Build history of the part. All positions in model axes, mm. A direction names the side the tool comes from. Give positions to 0.01 mm unless a question says otherwise; leave off trailing zeros. Loops run counter-clockwise (first coordinate to the right, second up) from the corner with the lowest first, then second, coordinate; pieces in that order, holes last. Notation, with made-up numbers: M 84,89.5 L 121,89.5 A20 cw 121,100.5 Z; hole C -1.75,-11 d9. An arc over 180 degrees is marked long. Put each result on its own line as item: value.
Autodesk Inventor part; units mm, degrees
ref_plane "作業平面1" through (-10, -78.5, 30.5) normal (0, 0, -1) x (0, 1, 0)
ref_plane "YZ Plane" through (0, 0, 0) normal (1, 0, 0) x (0, 1, 0)
ref_plane "XZ Plane" through (0, 0, 0) normal (0, 1, 0) x (-1, 0, 0)
sketch "スケッチ1" plane through (0, 0, 0) normal (0, 0, 1) x (1, 0, 0)
  circle A0 centre (7, -1.5) radius 1.1
  circle A1 centre (-7, -1.5) radius 1.1
  arc A2 (-7, 6.5) -> (-4, 3.5) centre (-4, 6.5) ccw
  line L0 (4, 3.5) -> (-4, 3.5)
  arc A3 (4, 3.5) -> (7, 6.5) centre (4, 6.5) ccw
  line L1 (7, 27.5) -> (7, 6.5)
  line L2 (-7, 6.5) -> (-7, 27.5)
  arc A4 (-4, 30.5) -> (-7, 27.5) centre (-4, 27.5) ccw
  line L3 (-4, 30.5) -> (4, 30.5)
  circle A5 centre (-7, 35.5) radius 1.1
  circle A6 centre (7, 35.5) radius 1.1
  circle A7 centre (-7, -1.5) radius 1.1
  line L4 (7, 27.5) -> (7, 6.5)
  arc A8 (4, 3.5) -> (7, 6.5) centre (4, 6.5) ccw
  line L5 (4, 3.5) -> (-4, 3.5)
  arc A9 (-7, 6.5) -> (-4, 3.5) centre (-4, 6.5) ccw
  line L6 (-7, 6.5) -> (-7, 27.5)
  arc A10 (-4, 30.5) -> (-7, 27.5) centre (-4, 27.5) ccw
  line L7 (-4, 30.5) -> (4, 30.5)
  arc A11 (7, 27.5) -> (4, 30.5) centre (4, 27.5) ccw
  circle A12 centre (7, -1.5) radius 1.1
  arc A13 (6, -30) -> (6.4, -31.2) centre (8, -30) ccw
  arc A14 (6.4, -40.8) -> (6.4, -31.2) centre (0, -36) ccw
  arc A15 (6.4, -40.8) -> (6, -42) centre (8, -42) ccw
  line L8 (6, -42) -> (6, -42.5)
  arc A16 (6, -42.5) -> (10, -42.5) centre (8, -42.5) ccw
  line L9 (10, -42.5) -> (10, 76.5)
  arc A17 (10, 76.5) -> (6, 76.5) centre (8, 76.5) ccw
  line L10 (6, 76.5) -> (6, 76)
  arc A18 (6, 76) -> (6.4, 74.8) centre (8, 76) ccw
  arc A19 (6.4, 65.2) -> (6.4, 74.8) centre (0, 70) ccw
  arc A20 (6.4, 65.2) -> (6, 64) centre (8, 64) ccw
  line L11 (6, 64) -> (6, 60.696)
  arc A21 (6, 60.696) -> (6.9906, 58.9694) centre (8, 60.696) ccw
  line L12 (6.9906, 58.9694) -> (6.9906, 52.6121)
  arc A22 (6.9906, 52.6121) -> (6, 50.8855) centre (8, 50.8855) ccw
  line L13 (6, 50.8855) -> (6, 45.5)
  arc A23 (3, 42.5) -> (6, 45.5) centre (3, 45.5) ccw
  line L14 (3, 42.5) -> (-8, 42.5)
  arc A24 (-8, 42.5) -> (-10, 40.5) centre (-8, 40.5) ccw
  line L15 (-10, 40.5) -> (-10, -6.5)
  arc A25 (-10, -6.5) -> (-8, -8.5) centre (-8, -6.5) ccw
  line L16 (-8, -8.5) -> (3, -8.5)
  arc A26 (6, -11.5) -> (3, -8.5) centre (3, -11.5) ccw
  line L17 (6, -11.5) -> (6, -16.8855)
  arc A27 (6, -16.8855) -> (6.9906, -18.6121) centre (8, -16.8855) ccw
  line L18 (6.9906, -18.6121) -> (6.9906, -24.9694)
  arc A28 (6.9906, -24.9694) -> (6, -26.696) centre (8, -26.696) ccw
  line L19 (6, -26.696) -> (6, -30)
  circle A29 centre (8, 76.5) radius 1.1
  circle A30 centre (-8, 40.5) radius 1.1
  circle A31 centre (-8, -6.5) radius 1.1
  circle A32 centre (8, -42.5) radius 1.1
  circle A33 centre (8, -6.5) radius 1.1
  circle A34 centre (8, 40.5) radius 1.1
  line L20 (10, 37.6) -> (-10, 37.6)
  line L21 (10, 17) -> (-10, 17) construction
  line L22 (10, -3.6) -> (-10, -3.6)
  point P0 (0, 0)
  point P1 (-10, -3.6)
  point P2 (10, -3.6)
  dimension "d0" = 1
ref_plane "作業平面1" through (-10, -78.5, 30.5) normal (0, 0, -1) x (0, 1, 0)
extrude "押し出し1" add sketch "スケッチ1" along normal up to surface (30.5 mm away) contours L22 L15 L20 L9
fillet "フィレット1" radius 4.25 4 edges at (10, 37.6, 15.25) (-10, 37.6, 15.25) (10, -3.6, 15.25) (-10, -3.6, 15.25)
properties part number "suzikai" material "ABS プラスチック"
Q1. Drop a flat-ended pin along its axis: pin 1 Ø3 at (x, y) = (7, -1.5) entering from +Z. Give the stop position or say it passes through.
Here are the results:
pin 1: z = 30.5
Q2. Mould opens along X. For faces 3 (the flat face through (0, 37.6, 15)), 4 (the cylindrical face through (-8.79, -2.32, 15.46)), 5 (the cylindrical face through (-6.1, 4.36, 15.04)), 6 (the flat face through (10, 17, 15)) say: pulls with the +X half, pulls with the -X half, needs draft (parallel to the pull), parting line crosses it, or undercut.
Here are the results:
face 3: needs draft
face 4: pulls with the -X half
face 5: undercut
face 6: pulls with the +X half
Q3. Slice it at A-A (x = 2.5). List the corners of the cut face in (y, z), and give its area (3 significant figures).
Here are the results:
outline: M -3.6,0 L 3.5,0 L 3.5,30.5 L -3.6,30.5 Z; M 30.5,0 L 37.6,0 L 37.6,30.5 L 30.5,30.5 Z
area: 433 mm²
Q4. Slice it at D-D (x = 6.5). List the corners of the cut face in (y, z).
Here are the results:
outline: M -3.53,0 L -2.48,0 L -2.48,30.5 L -3.53,30.5 Z; M -0.52,0 L 4.84,0 L 4.84,30.5 L -0.52,30.5 Z; M 29.16,0 L 34.52,0 L 34.52,30.5 L 29.16,30.5 Z; M 36.48,0 L 37.53,0 L 37.53,30.5 L 36.48,30.5 Z
Q5. Probe line 1 (X direction, y = 17.5, z = 25); line 2 (X direction, y = -1, z = 22); line 3 (Y direction, x = -8, z = 20). List the from-to ranges inside material, lowest first. Write a range as from..to.
Here are the results:
line 1: -10..-7, 7..10
line 2: -9.67..-7.98, -6.02..6.02, 7.98..9.67
line 3: -2.96..-1.96, -1.04..35.04, 35.96..36.96
Q6. Slice it at C-C (y = 4.5). List the corners of the cut face in (x, z), and give its area (3 significant figures).
Here are the results:
outline: M -10,0 L -6.24,0 L -6.24,30.5 L -10,30.5 Z; M 6.24,0 L 10,0 L 10,30.5 L 6.24,30.5 Z
area: 230 mm²
Q7. Slice it at B-B (z = 7). List the corners of the cut face in (x, y), and give its area (3 significant figures).
Here are the results:
outline: M -10,0.65 A4.25 ccw -5.75,-3.6 L 5.75,-3.6 A4.25 ccw 10,0.65 L 10,33.35 A4.25 ccw 5.75,37.6 L -5.75,37.6 A4.25 ccw -10,33.35 Z; hole C -7,-1.5 d2.2; hole C -7,35.5 d2.2; hole M -7,6.5 A3 ccw -4,3.5 L 4,3.5 A3 ccw 7,6.5 L 7,27.5 A3 ccw 4,30.5 L -4,30.5 A3 ccw -7,27.5 Z; hole C 7,-1.5 d2.2; hole C 7,35.5 d2.2
area: 423 mm²
Q8. Tool access for faces 1 (the cylindrical face through (8.72, -2.39, 15.46)), 2 (the cylindrical face through (-6.14, 29.6, 15.04)): list every direction of +Z, -Z, +X, -X, +Y, -Y with a clear straight run to the whole face (end or side of a thin tool).
Here are the results:
face 1: +Z, -Z, +X, -Y
face 2: +Z, -Z
